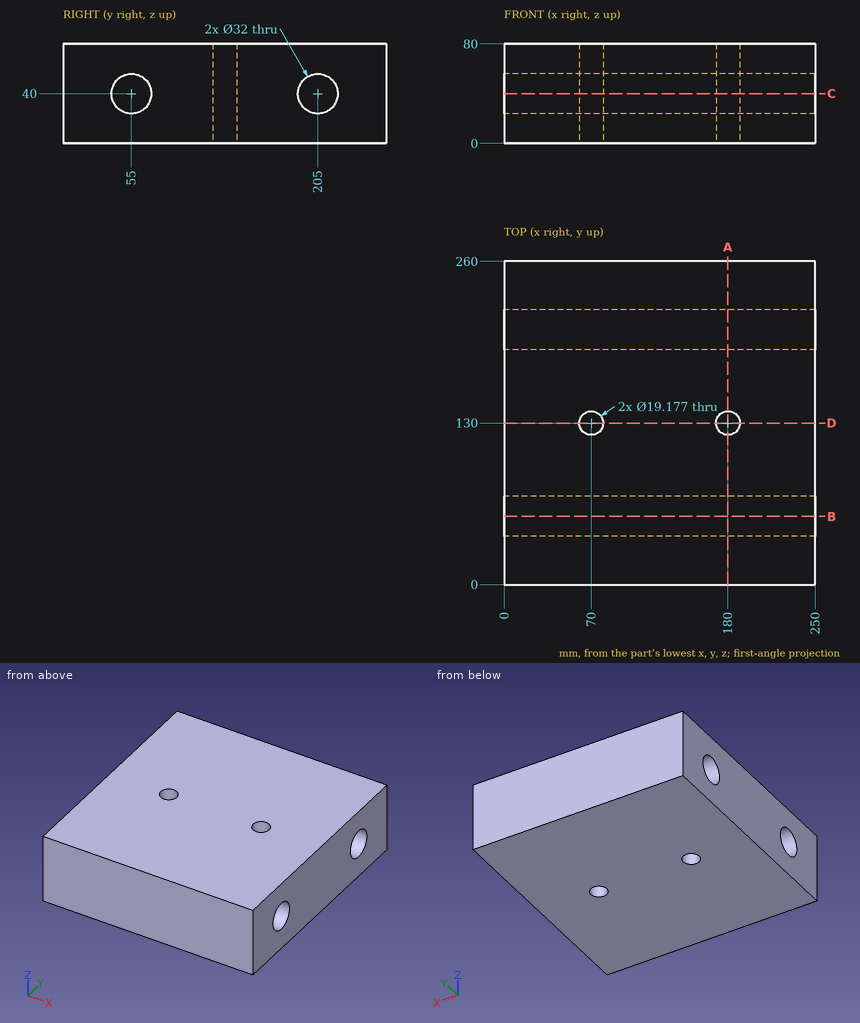
Study the drawing (mm; zero at the part's minimum x, y, z) and answer. Round coordinates to 2 decimals unless told otherwise and drop trailing zeros. Write each loop counter-clockwise with the first axis right and the second up, starting at its lowest first coordinate (ties: lowest second). Pieces come first, ordered by that corner, then holes. Notation, with made-up numbers: (-21.75, -19) - (30.25, -19) arc R10 ccw to (30.25, -8) - close; hole circle Ø4 at (-4, -12). An arc over 180 degrees is marked (long way). Use a Markdown table: item, result. Add a question column.
1. The part is cut by section B-B (y = 55). Write down the section's boundary in (x, z), and give its area (3 significant figures).
2. Flat-ended cylindrical pins translate along their axes: P1, Ø11.5, axis at x = 70, y = 130, coming from the -Z side; P2, Ø8, axis at y = 49.5, z = 13.5, coming from the -X side. Find the tip coordinate at first contact, or state that the pin passes through.
3. The part is cut by section D-D (y = 130). Write down the section's boundary in (x, z).
4. Consider line 1 (Y direction, x = 169, z = 40); line 2 (X direction, y = 130, z = 26.5); line 3 (Z direction, x = 124, y = 205). Determine where each line is inside the solid, lowest interval first.
5. The part is cut by section A-A (x = 180). Write down the section's boundary in (y, z).
6. The part is cut by section C-C (z = 40). Write down the section's boundary in (x, y), and give its area (3 significant figures).
Reported:
| question | item | result |
|---|---|---|
| 1 | outline | (0, 0) - (250, 0) - (250, 24) - (0, 24) - close; (0, 56) - (250, 56) - (250, 80) - (0, 80) - close |
| 1 | area | 12,000 mm^2 |
| 2 | P1 | through |
| 2 | P2 | x = 0 |
| 3 | outline | (0, 0) - (60.41, 0) - (60.41, 80) - (0, 80) - close; (79.59, 0) - (170.41, 0) - (170.41, 80) - (79.59, 80) - close; (189.59, 0) - (250, 0) - (250, 80) - (189.59, 80) - close |
| 4 | line 1 | 0 to 39, 71 to 189, 221 to 260 |
| 4 | line 2 | 0 to 60.41, 79.59 to 170.41, 189.59 to 250 |
| 4 | line 3 | 0 to 24, 56 to 80 |
| 5 | outline | (0, 0) - (120.41, 0) - (120.41, 80) - (0, 80) - close; (139.59, 0) - (260, 0) - (260, 80) - (139.59, 80) - close; hole circle Ø32 at (55, 40); hole circle Ø32 at (205, 40) |
| 6 | outline | (0, 0) - (250, 0) - (250, 39) - (0, 39) - close; (0, 71) - (250, 71) - (250, 189) - (0, 189) - close; (0, 221) - (250, 221) - (250, 260) - (0, 260) - close; hole circle Ø19.18 at (70, 130); hole circle Ø19.18 at (180, 130) |
| 6 | area | 48,400 mm^2 |
